```python
from build123d import *

# Parameters (mm, degrees)
SKETCH1_R                                   = 18.009689256
EXTRUDE1_DEPTH                              = 50.8
EXTRUDE2_REACH                              = 141.193
EXTRUDE2_END_RADIUS                         = 23.015630095
SKETCH3_OUTSIDE_W                           = 146.071
SKETCH3_OUTSIDE_H                           = 80.638
EXTRUDE3_DEPTH                              = 1.016
F_2_64_TAPPED_HOLE1_D                       = 1.778
F_2_64_TAPPED_HOLE1_DEPTH                   = 5.588
F_2_64_TAPPED_HOLE1_CBORE_D                 = 2.1844
F_2_64_TAPPED_HOLE1_CBORE_DEPTH             = 4.318
F_2_64_TAPPED_HOLE1_TIP                     = 0.53416509
CBORE_FOR_8_BINDING_HEAD_MACHINE_SC_2_COUNT = 2
CBORE_FOR_8_BINDING_HEAD_MACHINE_SC_2_PITCH = 32.054466339
CBORE_FOR_8_BINDING_HEAD_MACHINE_SC_3_COUNT = 2
CBORE_FOR_8_BINDING_HEAD_MACHINE_SC_3_PITCH = 89.830079482
CBORE_FOR_8_BINDING_HEAD_MACHINE_SC_4_COUNT = 2
CBORE_FOR_8_BINDING_HEAD_MACHINE_SC_4_PITCH = 95.377838055


with BuildPart() as part:
    # Sketch1 → Extrude1 (new body)
    with BuildSketch(Plane.XY):
        with BuildLine():
            Line((81.131890127, 9.040147783), (113.057520064, 9.040147783))
            ThreePointArc((113.057520064, 9.040147783), (115.302584094, 8.110211814), (116.232520064, 5.865147783))
            Line((116.232520064, 5.865147783), (116.232520064, 0))
            Line((116.232520064, 0), (116.232520064, -5.849507389))
            Line((116.232520064, -5.849507389), (105.291133005, -5.849507389))
            Line((105.291133005, -5.849507389), (105.291133005, 0))
            Line((105.291133005, 0), (10.941387059, 0))
            Line((10.941387059, 0), (10.941387059, -5.849507389))
            Line((10.941387059, -5.849507389), (0, -5.849507389))
            Line((0, -5.849507389), (0, 0))
            Line((0, 0), (0, 5.865147783))
            ThreePointArc((0, 5.865147783), (0.92993597, 8.110211814), (3.175, 9.040147783))
            Line((3.175, 9.040147783), (35.100629937, 9.040147783))
            Line((35.100629937, 9.040147783), (35.100629937, 25.900492611))
            ThreePointArc((35.100629937, 25.900492611), (58.116260032, 48.916122706), (81.131890127, 25.900492611))
            Line((81.131890127, 25.900492611), (81.131890127, 9.040147783))
        make_face()
        with Locations((58.116260032, 25.900492611)):
            Circle(SKETCH1_R, mode=Mode.SUBTRACT)
    extrude(amount=-EXTRUDE1_DEPTH)

    # Extrude2: up to this cylinder (the profile starts outside it)
    extrude2_end = Plane(origin=(58.116260032, 25.900492611, -25.4), z_dir=(0, 0, 1)) * Cylinder(EXTRUDE2_END_RADIUS, 329.41726019, mode=Mode.PRIVATE)
    # Sketch2 → Extrude2 (add, up to the surface)
    with BuildSketch(Plane(origin=(0, 51.456122706, 0), x_dir=(-1, 0, 0), z_dir=(0, 1, 0)), mode=Mode.PRIVATE) as extrude2_sk1:
        with BuildLine():
            Line((-62.33707365, -10.295164467), (-53.895446414, -10.295164467))
            ThreePointArc((-53.895446414, -10.295164467), (-52.81781568, -10.741533732), (-52.371446414, -11.819164467))
            Line((-52.371446414, -11.819164467), (-52.371446414, -38.980835533))
            ThreePointArc((-52.371446414, -38.980835533), (-52.81781568, -40.058466268), (-53.895446414, -40.504835533))
            Line((-53.895446414, -40.504835533), (-62.33707365, -40.504835533))
            ThreePointArc((-62.33707365, -40.504835533), (-63.414704384, -40.058466268), (-63.86107365, -38.980835533))
            Line((-63.86107365, -38.980835533), (-63.86107365, -11.819164467))
            ThreePointArc((-63.86107365, -11.819164467), (-63.414704384, -10.741533732), (-62.33707365, -10.295164467))
        make_face()
    extrude2_tool1 = extrude(extrude2_sk1.sketch, amount=-EXTRUDE2_REACH, mode=Mode.PRIVATE) - extrude2_end
    add(extrude2_tool1.solids().sort_by_distance((58.11626, 51.456123, -25.4))[0])

    # Sketch3 outside → Extrude3 (cut)
    # profile 1 of 2: a face of its own
    with BuildSketch(Plane(origin=(0, 51.456122706, 0), x_dir=(-1, 0, 0), z_dir=(0, 1, 0))):
        with Locations((-58.1165, -25.4)):
            Rectangle(SKETCH3_OUTSIDE_W, SKETCH3_OUTSIDE_H)
        with BuildLine():
            Line((-63.86107365, -11.819164467), (-63.86107365, -38.980835533))
            ThreePointArc((-63.86107365, -38.980835533), (-63.414704384, -40.058466268), (-62.33707365, -40.504835533))
            Line((-62.33707365, -40.504835533), (-53.895446414, -40.504835533))
            ThreePointArc((-53.895446414, -40.504835533), (-52.81781568, -40.058466268), (-52.371446414, -38.980835533))
            Line((-52.371446414, -38.980835533), (-52.371446414, -11.819164467))
            ThreePointArc((-52.371446414, -11.819164467), (-52.81781568, -10.741533732), (-53.895446414, -10.295164467))
            Line((-53.895446414, -10.295164467), (-62.33707365, -10.295164467))
            ThreePointArc((-62.33707365, -10.295164467), (-63.414704384, -10.741533732), (-63.86107365, -11.819164467))
        make_face(mode=Mode.SUBTRACT)
    # profile 2 of 2: a face of its own
    with BuildSketch(Plane(origin=(0, 51.456122706, 0), x_dir=(-1, 0, 0), z_dir=(0, 1, 0))):
        with BuildLine():
            Line((-54.657446414, -11.819164467), (-61.57507365, -11.819164467))
            ThreePointArc((-61.57507365, -11.819164467), (-62.113889017, -12.0423491), (-62.33707365, -12.581164467))
            Line((-62.33707365, -12.581164467), (-62.33707365, -38.218835533))
            ThreePointArc((-62.33707365, -38.218835533), (-62.113889017, -38.7576509), (-61.57507365, -38.980835533))
            Line((-61.57507365, -38.980835533), (-54.657446414, -38.980835533))
            ThreePointArc((-54.657446414, -38.980835533), (-54.118631047, -38.7576509), (-53.895446414, -38.218835533))
            Line((-53.895446414, -38.218835533), (-53.895446414, -12.581164467))
            ThreePointArc((-53.895446414, -12.581164467), (-54.118631047, -12.0423491), (-54.657446414, -11.819164467))
        make_face()
    extrude(amount=-EXTRUDE3_DEPTH, mode=Mode.SUBTRACT)

    # #2-64 Tapped Hole1
    with Locations(Plane(origin=(0, 50.440122706, 0), x_dir=(-1, 0, 0), z_dir=(0, 1, 0))):
        with Locations((-58.116260032, -17.825633593), (-58.116260032, -32.974366407)):
            CounterBoreHole(F_2_64_TAPPED_HOLE1_D / 2, F_2_64_TAPPED_HOLE1_CBORE_D / 2, F_2_64_TAPPED_HOLE1_CBORE_DEPTH, depth=F_2_64_TAPPED_HOLE1_DEPTH)
            with Locations((0, 0, -(F_2_64_TAPPED_HOLE1_DEPTH + F_2_64_TAPPED_HOLE1_TIP / 2))):  # 118° drill point
                Cone(0, F_2_64_TAPPED_HOLE1_D / 2, F_2_64_TAPPED_HOLE1_TIP, mode=Mode.SUBTRACT)

    # Sketch8 → CBORE for #8 Binding Head Machine Screw1 (revolve, cut)
    with BuildSketch(Plane(origin=(103.031299773, 9.040147783, -9.372766831), x_dir=(0, 0, 1), z_dir=(1, 0, 0))):
        Polygon((0, 0), (0, 14.889655172), (2.2479, 14.889655172), (2.2479, 2.667), (4.7625, 2.667), (4.7625, 0.635), (5.3975, 0), align=None)
    cbore_for_8_binding_head_machine_screw1 = revolve(axis=Axis((103.031299773, 15.390147783, -9.372766831), (0, -1, 0)), mode=Mode.SUBTRACT)

    # CBORE for _8 Binding Head Machine Sc 2: CBORE for #8 Binding Head Machine Screw1 ×2
    with Locations(*[(0, 0, -i * CBORE_FOR_8_BINDING_HEAD_MACHINE_SC_2_PITCH) for i in range(1, CBORE_FOR_8_BINDING_HEAD_MACHINE_SC_2_COUNT)]):
        add(cbore_for_8_binding_head_machine_screw1, mode=Mode.SUBTRACT)

    # CBORE for _8 Binding Head Machine Sc 3: CBORE for #8 Binding Head Machine Screw1 ×2
    with Locations(*[(-i * CBORE_FOR_8_BINDING_HEAD_MACHINE_SC_3_PITCH, 0, 0) for i in range(1, CBORE_FOR_8_BINDING_HEAD_MACHINE_SC_3_COUNT)]):
        add(cbore_for_8_binding_head_machine_screw1, mode=Mode.SUBTRACT)

    # CBORE for _8 Binding Head Machine Sc 4: CBORE for #8 Binding Head Machine Screw1 ×2
    with Locations(*[Vector(-0.941833882106029, 0, -0.33607876832237826) * (i * CBORE_FOR_8_BINDING_HEAD_MACHINE_SC_4_PITCH) for i in range(1, CBORE_FOR_8_BINDING_HEAD_MACHINE_SC_4_COUNT)]):
        add(cbore_for_8_binding_head_machine_screw1, mode=Mode.SUBTRACT)


solid = part.part
```
CAD build for the part. Positions are in the model's coordinates, mm. A direction names the side the tool comes from. Give positions to 0.01 mm unless a question says otherwise; leave off trailing zeros. Loops run counter-clockwise (first coordinate to the right, second up) from the corner with the lowest first, then second, coordinate; pieces in that order, holes last. Notation, with made-up numbers: (76.5, -38.5) - (122.5, -38.5) arc R8 ccw to (122.5, -24.5) - close; hole circle Ø4 at (-7, -10). An arc over 180 degrees is marked (long way). Put each result on its own line as item: value.
Q1. Slice it at B-B (y = 17.5). Give the cut face in (x, z).
Filled in:
outline: (35.1, -50.8) - (42.19, -50.8) - (42.19, 0) - (35.1, 0) - close; (74.05, -50.8) - (81.13, -50.8) - (81.13, 0) - (74.05, 0) - close
Q2. Slice it at C-C (x = 44). Give the cut face in (y, z), plus the area to 3 significant figures.
Filled in:
outline: (0, -50.8) - (14.72, -50.8) - (14.72, 0) - (0, 0) - close; (37.08, -50.8) - (44.08, -50.8) - (44.08, 0) - (37.08, 0) - close
area: 1,100 mm²
Q3. Mould opens along X. For faces 1 (the face through (65.5, 47.7, -25)), 2 (the face through (6, -5.85, -25)), 3 (the face through (98.31, 7.4, -9.99)) say: pulls with the +X half, pulls with the -X half, needs draft (parallel to the pull), parting line crosses it, or undercut.
Filled in:
face 1: parting line crosses it
face 2: needs draft
face 3: undercut
Q4. Flat gauge pins, fed straight in: pin 1 (1.5 mm diameter, centred on x = 83.5, z = -27.5, fed in from +Y); pin 2 (8.5 mm diameter, centred on y = 19.5, z = -32.5, fed in from -X); pin 3 (1.7 mm diameter, centred on x = 58.12, z = -32.97, fed in from -Y); pin 4 (2.5 mm diameter, centred on x = 13.2, z = -9.37, fed in from -Y). Where does each tip first touch, or does it go through?
Filled in:
pin 1: stops at y = 9.04
pin 2: stops at x = 35.1
pin 3: stops at y = 0
pin 4: passes through
Q5. Slice it at D-D (x = 77.5). Give the cut face in (y, z).
Filled in:
outline: (0, -50.8) - (38.31, -50.8) - (38.31, 0) - (0, 0) - close
Q6. Probe line 1 along X through (y, z) = (5.5, -39.5); line 2 along Y through (x, z) = (105.5, -16); line 3 along X through (y, z) = (6, -38.5). List the from-to ranges inside material, lowest first.
Filled in:
line 1: x = 0 to 12.04, 14.36 to 101.87, 104.19 to 116.23
line 2: y = -5.85 to 9.04
line 3: x = 0 to 116.23
Q7. Tool access for faces 4 (the face through (11.771, 7.403, -36.885)), 5 (the face through (97, 9.04, -25)), 6 (the face through (74.75, 19, -25.04)), 7 (the face through (105.291, -3, -25)): list every direction of +Z, -Z, +X, -X, +Y, -Y with a clear straight run to the whole face (end or side of a thin tool).
Filled in:
face 4: +Y
face 5: +Z, -Z, +X, +Y
face 6: +Z, -Z
face 7: +Z, -Z, -Y
